Verification items for the finished model (mm, model axes). Round coordinates to 2 decimals unless told otherwise and drop trailing zeros. Write each loop counter-clockwise with the first axis right and the second up, starting at its lowest first coordinate (ties: lowest second). Pieces come first, ordered by that corner, then holes. Notation, with made-up numbers: (58, -6) - (97, -6) arc R16 cw to (97, 9) - close; hole circle Ø1 at (-20.75, 71). An arc over 180 degrees is marked (long way). Answer as a JSON object with one key per item and string values. Group by question number.
1) Go/stop test with flat-tipped pins: pin 1 Ø2.5 at (x, y) = (-120, 238.66) entering from -Z; pin 2 Ø2.5 at (x, z) = (9, 1.5) entering from -Y. Record where each tip stops, or that it passes through.
2) Section check A-A (x = -48.5). Enter the section's corners in (y, z), then the cut area to 3 significant figures.
3) Section check B-B (z = 1.6). State how many separate pieces and enclosed holes the cut face has, then the cut area to 3 significant figures.
4) Thickness scan on line 1 (X direction, y = 230, z = 3.35); line 2 (Y direction, x = -125, z = 3.3); line 3 (Y direction, x = -130, z = 1.2). Record the ranges inside material, lowest first.
```python
from build123d import *

# Parameters (mm, degrees)
SKETCH1_R           = 3.292374312
SKETCH1_R_2         = 3.294421934
SKETCH1_R_3         = 3.163533699
SKETCH1_R_4         = 1.5
SKETCH1_R_5         = 4.7625
BOSS_EXTRUDE1_DEPTH = 4.7625


with BuildPart() as part:
    # Sketch1 → Boss-Extrude1 (new body)
    with BuildSketch(Plane.XY):
        Polygon((-436.816755826, -147.994392447), (-436.816755826, -169.55039994), (-596.816755826, -169.55039994), (-596.816755826, -150), (-596.816755826, 320), (215.080766979, 320), (215.080766979, -147.994392447), align=None)
        with Locations(Location((-589.375723826, -142.5578, 0), (0, 0, 180))):
            Circle(SKETCH1_R, mode=Mode.SUBTRACT)
        with Locations(Location((207.642212326, -142.5578, 0), (0, 0, 180))):
            Circle(SKETCH1_R, mode=Mode.SUBTRACT)
        with Locations(Location((207.642212326, 312.5578, 0), (0, 0, 180))):
            Circle(SKETCH1_R_2, mode=Mode.SUBTRACT)
        with Locations(Location((-589.375723826, 312.5578, 0), (0, 0, 180))):
            Circle(SKETCH1_R_3, mode=Mode.SUBTRACT)
        with Locations(Location((-135, 230, 0), (0, 0, 180))):
            Circle(SKETCH1_R_4, mode=Mode.SUBTRACT)
        with Locations(Location((-130, 238.660254038, 0), (0, 0, 180))):
            Circle(SKETCH1_R_4, mode=Mode.SUBTRACT)
        with Locations(Location((-120, 238.660254038, 0), (0, 0, 180))):
            Circle(SKETCH1_R_4, mode=Mode.SUBTRACT)
        with Locations(Location((-115, 230, 0), (0, 0, 180))):
            Circle(SKETCH1_R_4, mode=Mode.SUBTRACT)
        with Locations(Location((-120, 221.339745962, 0), (0, 0, 180))):
            Circle(SKETCH1_R_4, mode=Mode.SUBTRACT)
        with Locations(Location((-130, 221.339745962, 0), (0, 0, 180))):
            Circle(SKETCH1_R_4, mode=Mode.SUBTRACT)
        with Locations(Location((-125, 230, 0), (0, 0, 180))):
            Circle(SKETCH1_R_5, mode=Mode.SUBTRACT)
        with BuildLine():
            Line((-475, -100), (-518.031074044, -125.74437106))
            Line((-518.031074044, -125.74437106), (-546.780363752, -149.55039994))
            Line((-546.780363752, -149.55039994), (-459.597813184, -149.55039994))
            Line((-459.597813184, -149.55039994), (-459.597813184, -125.74437106))
            add(Edge.make_bspline(
                [(-459.597813184, -125.74437106), (-458.129207209, -124.865742348), (-455.185829054, -123.081513508), (-449.471359557, -119.524654219), (-442.555549408, -115.046151368), (-434.636214281, -109.639746192), (-424.556425744, -102.386073958), (-412.829398694, -93.24529863), (-400.055778993, -82.1905419), (-388.486450966, -71.092190732), (-374.537420018, -56.304576734), (-359.620141336, -37.979207276), (-344.890774823, -16.767556206), (-332.340078528, 3.245699555), (-321.055163892, 21.796443272), (-310.225956981, 38.664819129), (-299.079604806, 53.834809894), (-286.812791685, 67.514642691), (-272.431751915, 80.088460877), (-257.652665703, 89.924055398), (-243.498210685, 97.442015492), (-231.565093385, 102.886615769), (-218.172694067, 108.112662921), (-203.190999217, 113.087836875), (-189.281720356, 116.996077726), (-177.243425929, 119.962936855), (-167.745823902, 122.104113686), (-157.766000623, 124.157339904), (-149.036898589, 125.791853127), (-141.799270328, 127.051772068), (-136.243143266, 127.972296195), (-131.502167372, 128.719120718), (-127.648712651, 129.303231945), (-125.690331117, 129.592450023), (-124.714693771, 129.734664734)],
                knots=[0, 0, 0, 0, 0.00777259, 0.01554518, 0.03109036, 0.04663554, 0.062180721, 0.093271081, 0.124361441, 0.155451801, 0.186542162, 0.248722882, 0.310903603, 0.373084323, 0.435265044, 0.497445764, 0.559626485, 0.621807206, 0.683987926, 0.746168647, 0.777259007, 0.808349367, 0.839439728, 0.870530088, 0.901620448, 0.917165628, 0.932710808, 0.948255989, 0.963801169, 0.971573759, 0.979346349, 0.987118939, 0.991005234, 0.994891529, 0.994891529, 0.994891529, 0.994891529], degree=3))
            ThreePointArc((-124.714693771, 129.734664734), (-77.172123272, 119.052933104), (-32.323699215, 100))
            Line((-32.323699215, 100), (81.77450832, 31.56416045))
            Line((81.77450832, 31.56416045), (140.88780849, 31.56416045))
            Line((140.88780849, 31.56416045), (177.923308763, 55.973921994))
            Line((177.923308763, 55.973921994), (161.413907899, 81.022668132))
            Line((161.413907899, 81.022668132), (131.890654865, 61.56416045))
            Line((131.890654865, 61.56416045), (90.97120992, 61.56416045))
            ThreePointArc((90.97120992, 61.56416045), (35.57180112, 96.520479224), (-21.701372103, 128.313911667))
            Line((-21.701372103, 128.313911667), (-25, 130))
            ThreePointArc((-25, 130), (-73.684930832, 149.383563894), (-125, 160))
            add(Edge.make_bspline(
                [(-475, -100), (-419.540575809, -66.820070684), (-329.590802121, 43.11603253), (-307.635554762, 134.287094016), (-125, 160)],
                knots=[0, 0, 0, 0, 0.312223899, 1, 1, 1, 1], degree=3))
        make_face(mode=Mode.SUBTRACT)
    extrude(amount=BOSS_EXTRUDE1_DEPTH)


solid = part.part
```
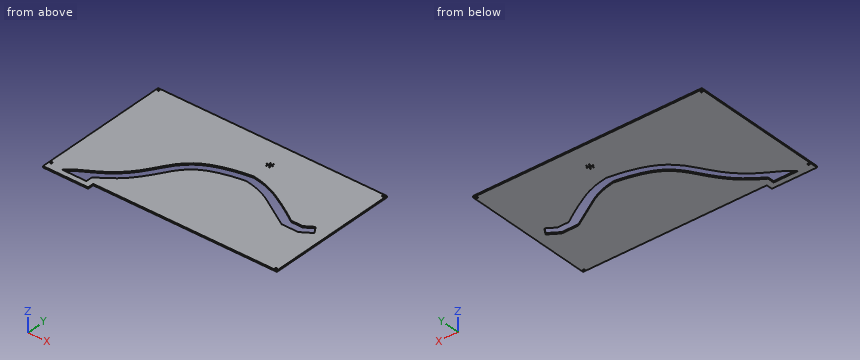
Returned:
{
 "1": {"pin 1": "through", "pin 2": "y = -147.99"},
 "2": {"outline": "(-147.99, 0) - (107.99, 0) - (107.99, 4.76) - (-147.99, 4.76) - close; (140.59, 0) - (320, 0) - (320, 4.76) - (140.59, 4.76) - close", "area": "2,070 mm2"},
 "3": {"separate pieces": "1", "enclosed holes": "12", "area": "357,000 mm2"},
 "4": {"line 1": "-596.82 to -136.5, -133.5 to -129.76, -120.24 to -116.5, -113.5 to 215.08", "line 2": "-147.99 to 129.69, 160 to 225.24, 234.76 to 320", "line 3": "-147.99 to 128.95, 159.28 to 219.84, 222.84 to 237.16, 240.16 to 320"}
}
